from build123d import *

# Parameters (mm, degrees)
EXTRUDE_1_DEPTH     = 17.75
CUT_EXTRUDE_1_DEPTH = 1
SKETCH_3_W          = 2.94
SKETCH_3_H          = 1
CUT_EXTRUDE_2_DEPTH = 6.5
CUT_EXTRUDE_3_DEPTH = 3.9
SKETCH_5_W          = 12.7
SKETCH_5_H          = 2.983573368
CUT_EXTRUDE_4_DEPTH = 1.4
SKETCH_6_W          = 12.7
SKETCH_6_H          = 2.983573368
CUT_EXTRUDE_5_DEPTH = 13.9
SKETCH_7_W          = 14.55
SKETCH_7_H          = 11.9
CUT_EXTRUDE_6_DEPTH = 3
EXTRUDE_2_DEPTH     = 0.5
EXTRUDE_3_DEPTH     = 0.5
EXTRUDE_4_DEPTH     = 2
CUT_EXTRUDE_7_DEPTH = 1
SKETCH_12_W         = 12.7
SKETCH_12_H         = 0.7
EXTRUDE_5_DEPTH     = 1.25
FILLET_1_R          = 1.5
EXTRUDE_6_DEPTH     = 0.95


with BuildPart() as part:
    # Эскиз1 → Бобышка-Вытянуть1 (new body)
    with BuildSketch(Plane(origin=(0, 0, 0), x_dir=(1, 0, 0), z_dir=(0, 1, 0))):
        with BuildLine():
            Line((-7.35, 2.75), (-7.35, 5.5))
            Line((-7.35, 5.5), (7.35, 5.5))
            Line((7.35, 5.5), (7.35, 2.75))
            Line((7.35, 2.75), (8.71, 1.55))
            Line((8.71, 1.55), (8.71, 0))
            ThreePointArc((8.71, 0), (0, 3.039347647), (-8.71, 0))
            Line((-8.71, 0), (-8.71, 1.55))
            Line((-8.71, 1.55), (-7.35, 2.75))
        make_face()
    extrude(amount=EXTRUDE_1_DEPTH)

    # Эскиз2 → Вырез-Вытянуть1 (cut)
    with BuildSketch(Plane(origin=(0, 17.75, 0), x_dir=(1, 0, 0), z_dir=(0, 1, 0))):
        with BuildLine():
            Line((8.71, 0.631840908), (8.71, 1.55))
            Line((8.71, 1.55), (7.35, 2.75))
            Line((7.35, 2.75), (7.35, 5.5))
            Line((7.35, 5.5), (-7.35, 5.5))
            Line((-7.35, 5.5), (-7.35, 2.75))
            Line((-7.35, 2.75), (-8.71, 1.55))
            Line((-8.71, 1.55), (-8.71, 0.631840908))
            ThreePointArc((-8.71, 0.631840908), (0, 3.539347647), (8.71, 0.631840908))
        make_face()
    extrude(amount=-CUT_EXTRUDE_1_DEPTH, mode=Mode.SUBTRACT)

    # Эскиз3 → Вырез-Вытянуть2 (cut, through all)
    with BuildSketch(Plane(origin=(0, 0, -5.5), x_dir=(-1, 0, 0), z_dir=(0, 0, -1))):
        with Locations((0, 17.25)):
            Rectangle(SKETCH_3_W, SKETCH_3_H)
    extrude(amount=-CUT_EXTRUDE_2_DEPTH, mode=Mode.SUBTRACT)

    # Эскиз4 → Вырез-Вытянуть3 (cut)
    with BuildSketch(Plane.XZ):
        with BuildLine():
            Line((-7.35, -2.75), (-7.35, -0.954778819))
            ThreePointArc((-7.35, -0.954778819), (-8.044178059, -0.497584831), (-8.71, 0))
            Line((-8.71, 0), (-8.71, -1.55))
            Line((-8.71, -1.55), (-7.35, -2.75))
        make_face()
        with BuildLine():
            Line((7.35, -2.75), (7.35, -0.954778819))
            ThreePointArc((7.35, -0.954778819), (8.044178059, -0.497584831), (8.71, 0))
            Line((8.71, 0), (8.71, -1.55))
            Line((8.71, -1.55), (7.35, -2.75))
        make_face()
    extrude(amount=-CUT_EXTRUDE_3_DEPTH, mode=Mode.SUBTRACT)

    # Эскиз5 → Вырез-Вытянуть4 (cut)
    with BuildSketch(Plane.XZ):
        with Locations((0, -3.008213316)):
            Rectangle(SKETCH_5_W, SKETCH_5_H)
    extrude(amount=-CUT_EXTRUDE_4_DEPTH, mode=Mode.SUBTRACT)

    # Эскиз6 → Вырез-Вытянуть5 (cut)
    with BuildSketch(Plane(origin=(0, 1.9, 0), x_dir=(-1, 0, 0), z_dir=(0, -1, 0))):
        with Locations((0, 3.008213316)):
            Rectangle(SKETCH_6_W, SKETCH_6_H)
    extrude(amount=-CUT_EXTRUDE_5_DEPTH, mode=Mode.SUBTRACT)

    # Эскиз7 → Вырез-Вытянуть6 (cut, through all)
    with BuildSketch(Plane(origin=(0, 0, -2), x_dir=(-1, 0, 0), z_dir=(0, 0, -1))):
        with Locations((0, 9.85)):
            Rectangle(SKETCH_7_W, SKETCH_7_H)
    extrude(amount=-CUT_EXTRUDE_6_DEPTH, mode=Mode.SUBTRACT)

    # Эскиз8 → Бобышка-Вытянуть2 (add)
    with BuildSketch(Plane.XZ.offset(-1.4)):
        with BuildLine():
            Line((-7.35, 0), (-4.825, 0))
            Line((-4.825, 0), (-4.325, -2.1))
            Line((-4.325, -2.1), (4.325, -2.1))
            Line((4.325, -2.1), (4.825, 0))
            Line((4.825, 0), (7.35, 0))
            Line((7.35, 0), (7.35, -0.954778819))
            ThreePointArc((7.35, -0.954778819), (0, -3.039347647), (-7.35, -0.954778819))
            Line((-7.35, -0.954778819), (-7.35, 0))
        make_face()
    extrude(amount=-EXTRUDE_2_DEPTH)

    # Эскиз9 → Бобышка-Вытянуть3 (add)
    with BuildSketch(Plane.XZ.offset(-1.4)):
        Polygon((-4.825, 0), (-5.122619048, 1.25), (-8.71, 1.25), (-7.35, 0), align=None)
        Polygon((4.825, 0), (5.122619048, 1.25), (8.71, 1.25), (7.35, 0), align=None)
    extrude(amount=-EXTRUDE_3_DEPTH)

    # Эскиз10 → Бобышка-Вытянуть4 (add)
    with BuildSketch(Plane(origin=(0, 1.9, 0), x_dir=(1, 0, 0), z_dir=(0, 1, 0))):
        with BuildLine():
            Line((-7.35, 0), (-8.71, -1.25))
            Line((-8.71, -1.25), (-6.35, -1.25))
            Line((-6.35, -1.25), (-6.35, 1.516426632))
            ThreePointArc((-6.35, 1.516426632), (-6.855753939, 1.24584747), (-7.35, 0.954778819))
            Line((-7.35, 0.954778819), (-7.35, 0))
        make_face()
        with BuildLine():
            Line((7.35, 0), (7.35, 0.954778819))
            ThreePointArc((7.35, 0.954778819), (6.855753939, 1.24584747), (6.35, 1.516426632))
            Line((6.35, 1.516426632), (6.35, -1.25))
            Line((6.35, -1.25), (8.71, -1.25))
            Line((8.71, -1.25), (7.35, 0))
        make_face()
    extrude(amount=EXTRUDE_4_DEPTH)

    # Эскиз11 → Вырез-Вытянуть7 (cut)
    with BuildSketch(Plane(origin=(0, 0, -5.5), x_dir=(-1, 0, 0), z_dir=(0, 0, -1))):
        with BuildLine():
            Line((-2.95, 3.15), (2.95, 3.15))
            ThreePointArc((2.95, 3.15), (3.6, 2.5), (2.95, 1.85))
            Line((2.95, 1.85), (-2.95, 1.85))
            ThreePointArc((-2.95, 1.85), (-3.6, 2.5), (-2.95, 3.15))
        make_face()
    extrude(amount=-CUT_EXTRUDE_7_DEPTH, mode=Mode.SUBTRACT)

    # Эскиз12 → Бобышка-Вытянуть5 (add)
    with BuildSketch(Plane.XY.offset(-4.5)):
        with Locations((0, 11.23)):
            Rectangle(SKETCH_12_W, SKETCH_12_H)
    extrude(amount=EXTRUDE_5_DEPTH)

    # Скругление1
    fillet_1_edges = [part.edges().sort_by_distance(p)[0] for p in [
        (-7.35, 8.375, -5.5),
        (7.35, 8.375, -5.5),
    ]]
    fillet(fillet_1_edges, radius=FILLET_1_R)

    # Эскиз13 → Бобышка-Вытянуть6 (add)
    with BuildSketch(Plane(origin=(0, 16.75, 0), x_dir=(1, 0, 0), z_dir=(0, 1, 0))):
        with BuildLine():
            Line((-1.47, 2.961958753), (-1.47, 1.8))
            Line((-1.47, 1.8), (1.47, 1.8))
            Line((1.47, 1.8), (1.47, 2.961958753))
            ThreePointArc((1.47, 2.961958753), (0, 3.039347647), (-1.47, 2.961958753))
        make_face()
    extrude(amount=-EXTRUDE_6_DEPTH)


solid = part.part
Model file for the job. Use its own axes, mm. A direction names the side the tool comes from. Give positions to 0.01 mm unless a question says otherwise; leave off trailing zeros. Loops run counter-clockwise (first coordinate to the right, second up) from the corner with the lowest first, then second, coordinate; pieces in that order, holes last. Notation, with made-up numbers: (87.25, 12.5) -> (110.25, 12.5) arc R27 ccw to (110.25, 34.5) -> close; hole circle Ø4 at (70, 4). An arc over 180 degrees is marked (long way). Use a Markdown table: item, result. Add a question column.
(1) Tool access for faces 4 (the flat face through (-7, 10, -2)), 5 (the cylindrical face through (5.232, 17.257, -2.562)), 6 (the flat face through (0, 1, -4.5)): list every direction of +Z, -Z, +X, -X, +Y, -Y with a clear straight run to the whole face (end or side of a thin tool).
(2) Mould opens along Y. For faces 1 (the cylindrical face through (6.863, 0.69, -1.242)), 2 (the flat face through (0, 1.4, -3)), 3 (the flat face through (-6.35, 9, -3)) say: +Y half, -Y half, draft (parallel to the pull), parting line (faces both ways), or undercut.
(3) Drop flat-ended pins along their axis: pin 1 Ø0.5 at (y, z) = (16, -2.5) entering from +X; pin 2 Ø0.6 at (x, y) = (-1, 1.5) entering from +Z; pin 3 Ø1.7 at (x, z) = (0, -3) entering from -Y. Give the stop position or say it passes through.
(4) Slice it at A-A on x = 0. List the corners of the cut face in (y, z), and give its area (3 significant figures).
(5) Wall check: line 1 along Y through (x, z) = (-3, -3.75); line 2 along Y through (x, z) = (2, -3); line 3 along Y through (x, z) = (-6, -3). Give the ranges that are in metal, low to high.
(6) Slice it at C-C on y = 2.5. List the corners of the cut face in (x, z).
(7) Slice it at B-B on z = -3.75. List the corners of the cut face in (x, y), and give its area (3 significant figures).
Filled sheet:
| question | item | result |
|---|---|---|
| 1 | face 4 | +Z |
| 1 | face 5 | -Z, +X, +Y |
| 1 | face 6 | +Z, -Y |
| 2 | face 1 | draft |
| 2 | face 2 | -Y half |
| 2 | face 3 | undercut |
| 3 | pin 1 | x = 7.92 |
| 3 | pin 2 | z = -2.1 |
| 3 | pin 3 | y = 1.4 |
| 4 | outline | (0, -5.5) -> (1.85, -5.5) -> (1.85, -4.5) -> (1.9, -4.5) -> (1.9, -2.1) -> (1.4, -2.1) -> (1.4, -4.5) -> (0, -4.5) -> close; (3.15, -5.5) -> (16.75, -5.5) -> (16.75, -1.8) -> (15.8, -1.8) -> (15.8, -4.5) -> (11.58, -4.5) -> (11.58, -3.25) -> (10.88, -3.25) -> (10.88, -4.5) -> (3.15, -4.5) -> close |
| 4 | area | 20.1 mm2 |
| 5 | line 1 | 1.4 to 1.9, 10.88 to 11.58, 15.8 to 16.75 |
| 5 | line 2 | 1.4 to 1.9, 15.8 to 17.75 |
| 5 | line 3 | 1.4 to 1.9, 15.8 to 16.75 |
| 6 | outline | (-8.71, 1.25) -> (-7.35, 0) -> (-7.35, -4) arc R1.5 ccw to (-5.85, -5.5) -> (-3.6, -5.5) -> (-3.6, -4.5) -> (-6.35, -4.5) -> (-6.35, 1.25) -> close; (3.6, -5.5) -> (5.85, -5.5) arc R1.5 ccw to (7.35, -4) -> (7.35, 0) -> (8.71, 1.25) -> (6.35, 1.25) -> (6.35, -4.5) -> (3.6, -4.5) -> close |
| 7 | outline | (-7.35, 0) -> (-6.35, 0) -> (-6.35, 1.4) -> (6.35, 1.4) -> (6.35, 0) -> (7.35, 0) -> (7.35, 16.75) -> (-7.35, 16.75) -> close; hole (-6.35, 1.9) -> (6.35, 1.9) -> (6.35, 10.88) -> (-6.35, 10.88) -> close; hole (-6.35, 11.58) -> (6.35, 11.58) -> (6.35, 15.8) -> (-6.35, 15.8) -> close |
| 7 | area | 60.8 mm2 |
